CAD build for the part. Positions are in the model's coordinates, mm. Face numbers are marked on the shaded views. A direction names the side the tool comes from. Round coordinates to 2 decimals unless told otherwise and drop trailing zeros. Loops run counter-clockwise (first coordinate to the right, second up) from the corner with the lowest first, then second, coordinate; pieces in that order, holes last. Notation, with made-up numbers: (11, -4.75) -> (47, -4.75) arc R24 ccw to (47, 18.25) -> close; hole circle Ø6 at (-30, 17). An arc over 180 degrees is marked (long way). Answer as CSV lines item,"result".
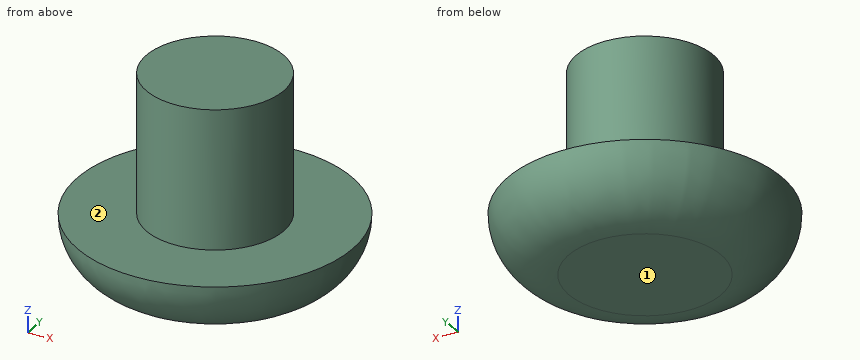
```python
from build123d import *

# Parameters (mm, degrees)
F0_R     = 11.43
F1_DEPTH = 5.08
F2_R     = 5.07999
F3_R     = 5.715
F4_DEPTH = 11.5697


# Not quite as in the source:
# - a fillet or chamfer is up to 0.001 mm smaller than in the source, because OpenCascade refuses the exact size


with BuildPart() as f1:
    # F0 (on Top) → F1 (new body)
    with BuildSketch(Plane.XY):
        Circle(F0_R)
    extrude(amount=F1_DEPTH)

    # F2 (radius 5.08 in the source; OpenCascade refuses exactly that, so slightly less here)
    f2_edges = [f1.edges().sort_by_distance(p)[0] for p in [
        (-11.43, 0, 0),
    ]]
    fillet(f2_edges, radius=F2_R)

    # F3 (on face) → F4 (join)
    with BuildSketch(Plane.XY.offset(5.08)):
        Circle(F3_R)
    extrude(amount=F4_DEPTH)


solid = f1.part
```
Q1. Slice it at C-C, the plane z = 12.5. Give the cut face in (x, y) (3 decimals), and give its area (3 significant figures).
Results:
outline,"circle Ø11.43 at (0, 0)"
area,"103 mm2"
Q2. Probe L1, parallel to X at y = 0.25, z = 9.25; L2, parallel to Y at x = -1.5, z = 5.5; L3, parallel to X at y = -1, z = 10. List the from-to ranges inside material, lowest first. Write a range as [from, to].
Results:
L1,"[-5.71, 5.71]"
L2,"[-5.51, 5.51]"
L3,"[-5.63, 5.63]"
Q3. Tool access for the marked faces 1 and 2: list every direction of +Z, -Z, +X, -X, +Y, -Y with a clear straight run to the whole face (end or side of a thin tool).
Results:
face 1,"-Z, +X, -X, +Y, -Y"
face 2,"+Z"
Q4. Drop flat-ended pins along their axis: pin 1 Ø1 at (x, z) = (-3.5, 14.5) entering from -Y; pin 2 Ø8 at (y, z) = (-7, 15) entering from +X; pin 3 Ø6 at (y, z) = (-9, 5) entering from -X. Give the stop position or say it passes through.
Results:
pin 1,"y = -4.86"
pin 2,"x = 4.86"
pin 3,"x = -9.73"
